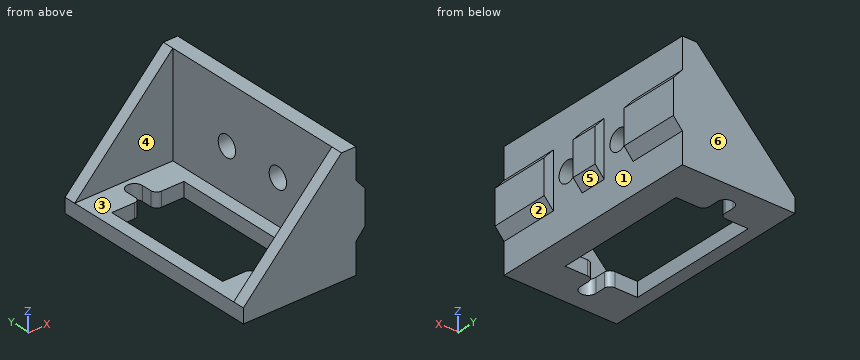
from build123d import *

# Parameters (mm, degrees)
PAD_DEPTH       = 37
PAD001_DEPTH    = 37
SKETCH002_W     = 17
SKETCH002_H     = 33
POCKET_DEPTH    = 17.5
SKETCH003_R     = 1.8
POCKET001_DEPTH = 21.061
SKETCH004_W     = 9.48
SKETCH004_H     = 6
POCKET002_DEPTH = 1.56
SKETCH005_W     = 12.5
SKETCH005_H     = 23
POCKET003_DEPTH = 2.501
POCKET004_DEPTH = 2.501
FILLET_R        = 1


with BuildPart() as part:
    # Sketch → Pad (new body)
    with BuildSketch(Plane.XZ):
        Polygon((-8.5, -7.5), (-8.5, -10), (11, -10), (11, -4.74), (12.56, -2.94), (12.56, 2.94), (11, 4.74), (11, 10), (8.5, 10), (8.5, -7.5), align=None)
    extrude(amount=PAD_DEPTH)

    # Sketch001 (on Face12 of Pad) → Pad001 (join)
    with BuildSketch(Plane.XZ.offset(37)):
        Polygon((8.5, 10), (-8.5, -7.5), (8.5, -7.5), align=None)
    extrude(amount=-PAD001_DEPTH)

    # Sketch002 (on Face8 of Pad001) → Pocket (cut)
    with BuildSketch(Plane(origin=(0, 0, 10), x_dir=(-1, 0, 0), z_dir=(0, 0, 1))):
        with Locations((0, 18.5)):
            Rectangle(SKETCH002_W, SKETCH002_H)
    extrude(amount=-POCKET_DEPTH, mode=Mode.SUBTRACT)

    # Sketch003 (on Face16 of Pocket) → Pocket001 (cut, through all)
    with BuildSketch(Plane(origin=(12.56, 0, 0), x_dir=(0, 0, 1), z_dir=(1, 0, 0))):
        with Locations((0, 23.786)):
            Circle(SKETCH003_R)
        with Locations((0, 13.214)):
            Circle(SKETCH003_R)
    extrude(amount=-POCKET001_DEPTH, mode=Mode.SUBTRACT)

    # Sketch004 (on Face16 of Pocket001) → Pocket002 (cut)
    with BuildSketch(Plane(origin=(12.56, 0, 0), x_dir=(0, 0, 1), z_dir=(1, 0, 0))):
        with Locations((0, 23.786)):
            Rectangle(SKETCH004_W, SKETCH004_H)
        with Locations((0, 13.214)):
            Rectangle(SKETCH004_W, SKETCH004_H)
    extrude(amount=-POCKET002_DEPTH, mode=Mode.SUBTRACT)

    # Sketch005 (on Face3 of Pocket002) → Pocket003 (cut, through all)
    with BuildSketch(Plane(origin=(0, 0, -7.5), x_dir=(-1, 0, 0), z_dir=(0, 0, 1))):
        with Locations((0, 18.5)):
            Rectangle(SKETCH005_W, SKETCH005_H)
    extrude(amount=-POCKET003_DEPTH, mode=Mode.SUBTRACT)

    # Sketch006 (on Face3 of Pocket003) → Pocket004 (cut, through all)
    with BuildSketch(Plane(origin=(0, 0, -7.5), x_dir=(-1, 0, 0), z_dir=(0, 0, 1))):
        with BuildLine():
            ThreePointArc((1.35, 32.75), (0, 34.1), (-1.35, 32.75))
            Line((-1.35, 32.75), (-1.35, 4.25))
            ThreePointArc((-1.35, 4.25), (0, 2.9), (1.35, 4.25))
            Line((1.35, 4.25), (1.35, 32.75))
        make_face()
    extrude(amount=-POCKET004_DEPTH, mode=Mode.SUBTRACT)

    # Fillet
    fillet_edges = [part.edges().sort_by_distance(p)[0] for p in [
        (1.35, -30, -8.75),
        (-1.35, -30, -8.75),
        (1.35, -7, -8.75),
        (-1.35, -7, -8.75),
    ]]
    fillet(fillet_edges, radius=FILLET_R)


solid = part.part
Design review of the part built by this model. Coordinates are the model's own, in mm. Face numbers are marked on the shaded views. A direction names the side the tool comes from. Round coordinates to 2 decimals unless told otherwise and drop trailing zeros. Write each loop counter-clockwise with the first axis right and the second up, starting at its lowest first coordinate (ties: lowest second). Pieces come first, ordered by that corner, then holes.
Item 1: Consider section B-B on y = -28. Give the boundary of the cut face in (x, z).
Item 2: Consider section D-D on z = -4. Give the boundary of the cut face in (x, y).
Item 3: Draft analysis for pull direction Y (two halves, no side actions). For the marked faces 4, 5 and 6, state which applies: released by +Y, released by -Y, zero draft, split by the parting line, or undercut.
Item 4: Consider section A-A on x = 0. Give the boundary of the cut face in (y, z).
Item 5: Consider section C-C on z = -0.75. Give the boundary of the cut face in (x, y), and give its area (3 significant figures).
Item 6: Wall thickness on L1, parallel to Y at x = 9.3, z = 0; L2, parallel to X at y = -21, z = 8; L3, parallel to Z at x = -4.25, y = -33: over which ranges is each line inside the solid? List them lowest first.
Item 7: For pin 1 Ø1.5 at (y, z) = (-21, -3) entering from -X; pin 2 Ø2 at (y, z) = (-23.786, 0) entering from -X; pin 3 Ø3 at (y, z) = (-16, 7) entering from +X; pin 4 Ø4 at (x, y) = (4.5, -20.5) entering from +Z, all flat-tipped, find the tip position at first contact; note any pin that passes through.
Item 8: For the marked faces 1, 2 and 3, list the 3-axis set-ups (+Z, -Z, +X, -X, +Y, -Y) from which the entire face can be reached by the end or side of a thin tool; tool diameter is ignored.
Check values:
1. outline: (-8.5, -10) - (-6.25, -10) - (-6.25, -7.5) - (-8.5, -7.5) - close; (6.25, -10) - (11, -10) - (11, -4.74) - (12.56, -2.94) - (12.56, 2.94) - (11, 4.74) - (11, 10) - (8.5, 10) - (8.5, -7.5) - (6.25, -7.5) - close
2. outline: (-5.1, -37) - (11.64, -37) - (11.64, -26.79) - (11, -26.79) - (11, -20.79) - (11.64, -20.79) - (11.64, -16.21) - (11, -16.21) - (11, -10.21) - (11.64, -10.21) - (11.64, 0) - (-5.1, 0) - (-5.1, -2) - (8.5, -2) - (8.5, -35) - (-5.1, -35) - close
3. face 4: undercut
3. face 5: zero draft
3. face 6: released by +Y
4. outline: (-37, -10) - (-34.1, -10) - (-34.1, -7.5) - (-35, -7.5) - (-35, 1.25) - (-37, 1.25) - close; (-2.9, -10) - (0, -10) - (0, 1.25) - (-2, 1.25) - (-2, -7.5) - (-2.9, -7.5) - close
5. outline: (-1.94, -37) - (12.56, -37) - (12.56, -26.79) - (11, -26.79) - (11, -25.42) - (8.5, -25.42) - (8.5, -35) - (-1.94, -35) - close; (-1.94, -2) - (8.5, -2) - (8.5, -11.58) - (11, -11.58) - (11, -10.21) - (12.56, -10.21) - (12.56, 0) - (-1.94, 0) - close; (8.5, -22.15) - (11, -22.15) - (11, -20.79) - (12.56, -20.79) - (12.56, -16.21) - (11, -16.21) - (11, -14.85) - (8.5, -14.85) - close
5. area: 157 mm2
6. L1: y = -37 to -25.59, -21.99 to -15.01, -11.41 to 0
6. L2: x = 8.5 to 11
6. L3: z = -10 to -7.5
7. pin 1: stops at x = 8.5
7. pin 2: passes through
7. pin 3: stops at x = 11
7. pin 4: stops at z = -7.5
8. face 1: +X
8. face 2: -Z, +X, +Y, -Y
8. face 3: +Z, -X
